Autodesk Inventor part; units mm, degrees
ref_plane "YZ Plane" through (0, 0, 0) normal (1, 0, 0) x (0, 1, 0)
ref_plane "XZ Plane" through (0, 0, 0) normal (0, 1, 0) x (-1, 0, 0)
ref_plane "XY Plane" through (0, 0, 0) normal (0, 0, 1) x (1, 0, 0)
sketch "Sketch2" plane through (0, 0, 0) normal (0, 0, 1) x (1, 0, 0)
  circle A0 centre (0, 0) radius 6.35
  dimension "d0" = 12.7
extrude "Extrusion1" add sketch "Sketch2" along normal mid plane 441.96
chamfer "Chamfer1" distance 1.27 angle 45 1 edges at (-6.35, 0, -220.98)
sketch "Sketch3" plane through (0, 0, 220.98) normal (0, 0, 1) x (1, 0, 0)
  line L0 (10.9985, 0) -> (5.4993, -9.525)
  line L1 (5.4993, -9.525) -> (-5.4993, -9.525)
  line L2 (-5.4993, -9.525) -> (-10.9985, 0)
  line L3 (-10.9985, 0) -> (-5.4993, 9.525)
  line L4 (-5.4993, 9.525) -> (5.4993, 9.525)
  line L5 (5.4993, 9.525) -> (10.9985, 0)
  point P0 (0, 0)
  point P1 (0, 0)
  dimension "d6" = 19.05
extrude "Extrusion2" add sketch "Sketch3" along normal blind 12.7
sketch "Sketch4" plane through (0, 0, 233.68) normal (0, 0, 1) x (1, 0, 0)
  circle A0 centre (0, 0) radius 6.35
extrude "Extrusion3" cut sketch "Sketch4" against normal blind 2.54
sketch "Sketch5" plane through (0, 0, 0) normal (1, 0, 0) x (0, 1, 0)
  line L0 (0, 233.68) -> (9.525, 233.68)
  line L1 (9.525, 233.68) -> (11.1053, 233.68) construction
  line L2 (13.1997, 229.5016) -> (7.8979, 234.7834)
  line L3 (7.8979, 234.7834) -> (10.6425, 234.7834)
  line L4 (10.6425, 234.7834) -> (13.1997, 229.5016)
  line L5 (0, -312.1327) -> (0, 325.9361)
  point P0 (0, 0)
revolve "Revolution1" cut sketch "Sketch5" angle 360 about axis through (0, 0, -10) along (0, 0, 1)
chamfer "Chamfer2" distance 1.27 angle 45 6 edges at (5.4993, 9.525, 226.3372) (10.9985, 0, 226.3372) (5.4993, -9.525, 226.3372) (-5.4993, -9.525, 226.3372) (-10.9985, 0, 226.3372) (-5.4993, 9.525, 226.3372)
properties part number "Through bolt"
Design review of the part built by this model. Coordinates are the model's own, in mm. A direction names the side the tool comes from. Round coordinates to 2 decimals unless told otherwise and drop trailing zeros. Loops run counter-clockwise (first coordinate to the right, second up) from the corner with the lowest first, then second, coordinate; pieces in that order, holes last. Notation, with made-up numbers: (26, -30) -> (69, -30) arc R11 cw to (69, -9) -> close; hole circle Ø9 at (-17.75, -39). An arc over 180 degrees is marked (long way). Use one line per item in the form item = value. Start each with the question number.
Q1. Machinability: for faces 4 (the face through (0, 0, 231.14)), 5 (the face through (-1.38, -6.2, 3.72)), 6 (the face through (4, -6, 233.68)), which of the approach directions +Z, -Z, +X, -X, +Y, -Y give a long, thin tool a straight path to every point of the face, cutting with its end or side? Answer none if there is none.
Q2. For pin 1 Ø2 at (x, y) = (-4, -5) entering from -Z; pin 2 Ø4 at (x, y) = (-1, 1.5) entering from +Z; pin 3 Ø1.5 at (y, z) = (-0.5, -145) entering from +X, all flat-tipped, find the tip position at first contact; note any pin that passes through.
Q3. Draft analysis for pull direction Y (two halves, no side actions). For faces 1 (the face through (-4.8, 4.4, 220.98)), 2 (the face through (8.22, 4.81, 226.99)), 3 (the face through (-1.38, -6.2, 232.43)), state which applies: +Y half, -Y half, draft (parallel to the pull), parting line (faces both ways), or undercut.
Q4. Wall thickness on line 1 along Y through (x, z) = (0, 232.2) (3 decimals); line 2 along Z through (x, y) = (5, 8); line 3 along Z through (x, y) = (-7, 3.25): over which ranges is each line inside the solid? List them lowest first. Write a range as [from, to].
Q5. We need section A-A on x = 0. Give the boundary of the cut face in (y, z) (3 decimals), then the cut area to 3 significant figures.
Q6. We need section B-B on z = -72. Give the boundary of the cut face in (x, y).
Calculated:
q1.face_4 = +Z
q1.face_5 = -Z
q1.face_6 = +Z, +X, -X, +Y, -Y
q2.pin_1 = -220.66
q2.pin_2 = 231.14
q2.pin_3 = 6.35
q3.face_1 = draft
q3.face_2 = +Y half
q3.face_3 = undercut
q4.line_1 = [-9.525, -6.35], [6.35, 9.525]
q4.line_2 = [220.98, 233.25]
q4.line_3 = [220.98, 233.68]
q5.outline = (-9.525, 220.98) -> (-6.35, 220.98) -> (-6.35, -219.71) -> (-5.08, -220.98) -> (5.08, -220.98) -> (6.35, -219.71) -> (6.35, 220.98) -> (9.525, 220.98) -> (9.525, 233.162) -> (9.005, 233.68) -> (6.35, 233.68) -> (6.35, 231.14) -> (-6.35, 231.14) -> (-6.35, 233.68) -> (-9.005, 233.68) -> (-9.525, 233.162) -> close
q5.area = 5,820 mm²
q6.outline = circle Ø12.7 at (0, 0)
